The listing builds one solid part. Answer for the finished solid, in the listing's coordinates (mm). Face numbers are marked on the shaded views. Round coordinates to 2 decimals unless told otherwise and drop trailing zeros. Write each loop counter-clockwise with the first axis right and the second up, starting at its lowest first coordinate (ties: lowest second). Pieces come first, ordered by that corner, then holes. Notation, with made-up numbers: (89.25, 62) - (109.25, 62) arc R14 cw to (109.25, 88) - close; hole circle Ø10 at (56.25, 73). An arc over 180 degrees is marked (long way). Use a Markdown table: item, result. Add a question column.
1) A cutting plane is placed at A-A (y = 11). Give the vertices of the cut face in (x, z), then the cut area to 3 significant figures.
2) Find the intervals of material crossed by probe 1 along Z at (x, y) = (38.5, 21); probe 2 along X at (y, z) = (28, -236); probe 3 along Y at (x, z) = (62, -30), in increasing order. Write a range as from..to.
3) A cutting plane is placed at C-C (z = -322). Give the vertices of the cut face in (x, y).
4) Determine the mould class of the marked faces 1 and 2 for opening direction X: +X half, -X half, draft (parallel to the pull), parting line (faces both ways), or undercut.
5) Each of these flat-tipped pins is pushed along its axis until it touches: P1, Ø3.5, axis at x = -5, y = 15.5, coming from the -Z side; P2, Ø2, axis at y = 20, z = -384.5, coming from the +X side; P3, Ø5.5, axis at y = 12, z = 4, coming from the -X side. Where does it stop, or does it pass through?
6) A cutting plane is placed at B-B (x = 23). Give the vertices of the cut face in (y, z), then the cut area to 3 significant figures.
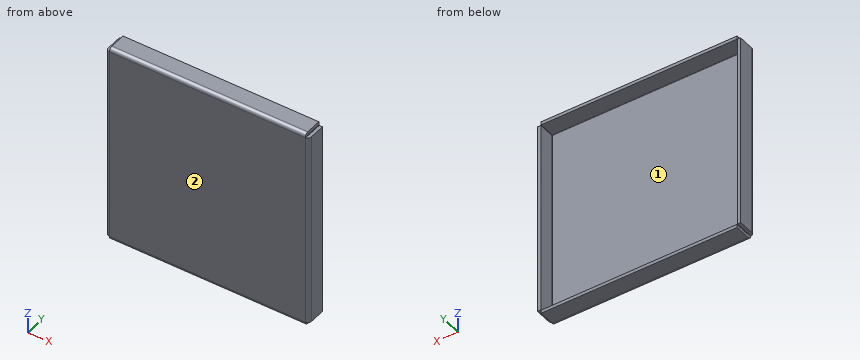
```python
from build123d import *

# Parameters (mm, degrees)
SKETCH1_W          = 381
SKETCH1_H          = 381
BASE_FLANGE1_DEPTH = 6.35
EDGE_FLANGE3_DEPTH = 381
EDGE_FLANGE4_DEPTH = 381
EDGE_FLANGE5_DEPTH = 381
EDGE_FLANGE6_DEPTH = 381


# Sheet-metal steps are written as plain solids
with BuildPart() as part:
    # Sketch1 → Base-Flange1 (new body)
    with BuildSketch(Plane(origin=(0, 0, 0), x_dir=(1, 0, 0), z_dir=(0, 1, 0))):
        with Locations((190.5, 190.5)):
            Rectangle(SKETCH1_W, SKETCH1_H)
    extrude(amount=-BASE_FLANGE1_DEPTH)

    # Edge-Flange3 section (across the edge) → Edge-Flange3 (add)
    with BuildSketch(Plane(origin=(-0.7366, 0, -381), x_dir=(1, 0, 0), z_dir=(0, 0, 1))):
        with BuildLine():
            Line((-6.35, 0.7366), (-6.35, 31.75))
            Line((-6.35, 31.75), (0, 31.75))
            Line((0, 31.75), (0, 0.7366))
            ThreePointArc((0, 0.7366), (0.215745145, 0.215745145), (0.7366, 0))
            Line((0.7366, 0), (0.7366, -6.35))
            ThreePointArc((0.7366, -6.35), (-4.274382916, -4.274382916), (-6.35, 0.7366))
        make_face()
    extrude(amount=EDGE_FLANGE3_DEPTH)

    # Edge-Flange4 section (across the edge) → Edge-Flange4 (add)
    with BuildSketch(Plane(origin=(381, 0, -381.7366), x_dir=(0, 0, 1), z_dir=(-1, 0, 0))):
        with BuildLine():
            Line((-6.35, 0.7366), (-6.35, 31.75))
            Line((-6.35, 31.75), (0, 31.75))
            Line((0, 31.75), (0, 0.7366))
            ThreePointArc((0, 0.7366), (0.215745145, 0.215745145), (0.7366, 0))
            Line((0.7366, 0), (0.7366, -6.35))
            ThreePointArc((0.7366, -6.35), (-4.274382916, -4.274382916), (-6.35, 0.7366))
        make_face()
    extrude(amount=EDGE_FLANGE4_DEPTH)

    # Edge-Flange5 section (across the edge) → Edge-Flange5 (add)
    with BuildSketch(Plane(origin=(0, 0, 0.7366), x_dir=(0, 0, -1), z_dir=(1, 0, 0))):
        with BuildLine():
            Line((-6.35, 0.7366), (-6.35, 31.75))
            Line((-6.35, 31.75), (0, 31.75))
            Line((0, 31.75), (0, 0.7366))
            ThreePointArc((0, 0.7366), (0.215745145, 0.215745145), (0.7366, 0))
            Line((0.7366, 0), (0.7366, -6.35))
            ThreePointArc((0.7366, -6.35), (-4.274382916, -4.274382916), (-6.35, 0.7366))
        make_face()
    extrude(amount=EDGE_FLANGE5_DEPTH)

    # Edge-Flange6 section (across the edge) → Edge-Flange6 (add)
    with BuildSketch(Plane(origin=(381.7366, 0, 0), x_dir=(-1, 0, 0), z_dir=(0, 0, -1))):
        with BuildLine():
            Line((-6.35, 0.7366), (-6.35, 31.75))
            Line((-6.35, 31.75), (0, 31.75))
            Line((0, 31.75), (0, 0.7366))
            ThreePointArc((0, 0.7366), (0.215745145, 0.215745145), (0.7366, 0))
            Line((0.7366, 0), (0.7366, -6.35))
            ThreePointArc((0.7366, -6.35), (-4.274382916, -4.274382916), (-6.35, 0.7366))
        make_face()
    extrude(amount=EDGE_FLANGE6_DEPTH)


solid = part.part
```
Entries:
| question | item | result |
|---|---|---|
| 1 | outline | (-7.09, -381) - (-0.74, -381) - (-0.74, 0) - (-7.09, 0) - close; (0, -388.09) - (381, -388.09) - (381, -381.74) - (0, -381.74) - close; (0, 0.74) - (381, 0.74) - (381, 7.09) - (0, 7.09) - close; (381.74, -381) - (388.09, -381) - (388.09, 0) - (381.74, 0) - close |
| 1 | area | 9,680 mm² |
| 2 | probe 1 | z = -388.09..-381.74, 0.74..7.09 |
| 2 | probe 2 | x = -7.09..-0.74, 381.74..388.09 |
| 2 | probe 3 | y = -6.35..0 |
| 3 | outline | (-7.09, 0.74) arc R7.09 ccw to (0, -6.35) - (381, -6.35) arc R7.09 ccw to (388.09, 0.74) - (388.09, 31.75) - (381.74, 31.75) - (381.74, 0.74) arc R0.74 cw to (381, 0) - (0, 0) arc R0.74 cw to (-0.74, 0.74) - (-0.74, 31.75) - (-7.09, 31.75) - close |
| 4 | face 1 | undercut |
| 4 | face 2 | draft |
| 5 | P1 | stops at z = -381 |
| 5 | P2 | stops at x = 381 |
| 5 | P3 | stops at x = 0 |
| 6 | outline | (-6.35, -381) arc R7.09 ccw to (0.74, -388.09) - (31.75, -388.09) - (31.75, -381.74) - (0.74, -381.74) arc R0.74 cw to (0, -381) - (0, 0) arc R0.74 cw to (0.74, 0.74) - (31.75, 0.74) - (31.75, 7.09) - (0.74, 7.09) arc R7.09 ccw to (-6.35, 0) - close |
| 6 | area | 2,890 mm² |
